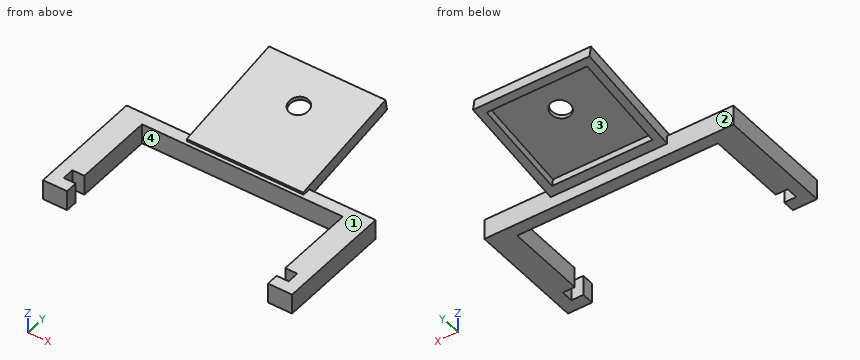
Autodesk Inventor part; units mm, degrees
ref_plane "YZ Plane" through (0, 0, 0) normal (1, 0, 0) x (0, 1, 0)
ref_plane "XZ Plane" through (0, 0, 0) normal (0, 1, 0) x (-1, 0, 0)
ref_plane "XY Plane" through (0, 0, 0) normal (0, 0, 1) x (1, 0, 0)
sketch "Esquisse1" plane through (0, 0, 0) normal (0, 0, 1) x (1, 0, 0)
  line L0 (-16.3902, 3.7398) -> (-19.3902, 3.7398)
  line L1 (-19.3902, 3.7398) -> (-19.3902, 0.7398)
  line L2 (-19.3902, 0.7398) -> (-16.3902, 0.7398)
  line L3 (-16.3902, 0.7398) -> (-16.3902, -2.2602)
  line L4 (-16.3902, -2.2602) -> (-22.3902, -2.2602)
  line L5 (-16.3902, 3.7398) -> (-16.3902, 23.7398)
  line L6 (33.6098, 23.7398) -> (33.6098, 3.7398)
  line L7 (33.6098, 3.7398) -> (36.6098, 3.7398)
  line L8 (36.6098, 3.7398) -> (36.6098, 0.7398)
  line L9 (36.6098, 0.7398) -> (33.6098, 0.7398)
  line L10 (33.6098, 0.7398) -> (33.6098, -2.2602)
  line L11 (33.6098, -2.2602) -> (39.6098, -2.2602)
  line L12 (-22.3902, 26.7398) -> (39.6098, 26.7398)
  line L13 (-16.3902, 23.7398) -> (33.6098, 23.7398)
  line L14 (-22.3902, 26.7398) -> (-22.3902, -2.2602)
  line L15 (39.6098, 26.7398) -> (39.6098, -2.2602)
  point P0 (0, 0)
  dimension "d0" = 56
  dimension "d1" = 3
  dimension "d2" = 3
  dimension "d3" = 3
  dimension "d4" = 3
  dimension "d5" = 20
  dimension "d6" = 20
  dimension "d7" = 50
  dimension "d8" = 3
  dimension "d9" = 6
  dimension "d10" = 6
  dimension "d11" = 3
  dimension "d12" = 3
extrude "Extrusion1" add sketch "Esquisse1" along normal blind 5
ref_plane "Plan de construction1" through (39.6098, 26.7398, 5) normal (0, 0.9848, 0.1736) x (-1, 0, 0)
sketch "Esquisse2" plane through (39.6098, 26.7398, 5) normal (0, 0.9848, 0.1736) x (-1, 0, 0)
  line L0 (45.5, -2) -> (16.5, -2)
  line L1 (16.5, -2) -> (16.5, 1)
  line L2 (16.5, 1) -> (45.5, 1)
  line L3 (45.5, 1) -> (45.5, -2)
  line L4 (0, 0) -> (62, 0)
  line L5 (0, -4.924) -> (0, 0)
  point P0 (39.6098, -0.2807)
  dimension "d16" = 29
  dimension "d17" = 3
  dimension "d18" = 1
  dimension "d23" = 16.5
extrude "Extrusion2" add sketch "Esquisse2" along normal blind 27 and the other way blind 2
sketch "Esquisse3" plane through (23.1098, 26.7398, 2.9691) normal (0, 0.1736, -0.9848) x (-1, 0, 0)
  line L0 (2, 25.3527) -> (27, 25.3527)
  line L1 (27, 25.3527) -> (27, 2.3527)
  line L2 (27, 2.3527) -> (2, 2.3527)
  line L3 (2, 2.3527) -> (2, 25.3527)
  line L4 (0, 27.3527) -> (29, 27.3527)
  line L5 (29, 0) -> (29, 27.3527)
  line L6 (-28.9, 0.3527) -> (57.9, 0.3527)
  line L7 (0, 0) -> (0, 27.3527)
  point P0 (23.1098, -26.8492)
  dimension "d24" = 2
  dimension "d25" = 2
  dimension "d26" = 2
  dimension "d27" = 2
extrude "Extrusion3" cut sketch "Esquisse3" against normal blind 2 contours L0 L1 L2 L3
sketch "Esquisse4" plane through (23.1098, 26.3925, 4.9388) normal (0, 0.1736, -0.9848) x (-1, 0, 0)
  circle A0 centre (14.3745, 17.1752) radius 2.5
  point P0 (23.1098, -26.8492)
  dimension "d30" = 5
extrude "Extrusion4" cut sketch "Esquisse4" against normal blind 10
properties part number "support_caméra"
Check sheet for the modelled part. Datum: model origin and axes. Units: mm. Face numbers are marked on the shaded views. Coordinates: 2 decimals unless noted, no trailing zeros. Loops run counter-clockwise (first coordinate to the right, second up) from the corner with the lowest first, then second, coordinate; pieces in that order, holes last. Notation, with made-up numbers: (-2.75, -19.75) -> (33.25, -19.75) arc R3 ccw to (33.25, -14.75) -> close; hole circle Ø10 at (-31.75, -26). An arc over 180 degrees is marked (long way). Write item = value, one per line. Start each with the question number.
1. Depth check by flat-ended pin: P1, Ø2.5, axis at x = 35, z = 3, coming from the +Y side; P2, Ø4, axis at y = 44, z = 7, coming from the -X side; P3, Ø2, axis at x = 11.5, y = 47, coming from the -Z side. Enter the tip coordinate at first touch or a pass-through.
2. Section check B-B on x = 20. Record the cut outline in (y, z), then the cut area to 3 significant figures.
3. Draft check along Y on the marked faces 1, 2, 3 and 4. Enter one of: released by +Y, released by -Y, zero draft, split by the parting line, or undercut.
4. Section check A-A on y = 2. Record the cut outline in (x, z).
5. Section check C-C on z = 1.5. Record the cut outline in (x, y).
6. Section check D-D on y = 48. Record the cut outline in (x, z).
7. Material ranges on line 1 (X direction, y = 50, z = 8.25); line 2 (X direction, y = 13, z = 2.25); line 3 (Y direction, x = -17, z = 3.5), recorded low to high.
Responses:
q1.P1 = 26.74
q1.P2 = -5.89
q1.P3 = 8.4
q2.outline = (23.74, 0) -> (26.74, 0) -> (26.74, 2.97) -> (29.06, 3.38) -> (28.71, 5.35) -> (51.36, 9.34) -> (51.71, 7.37) -> (53.68, 7.72) -> (53.16, 10.67) -> (24.6, 5.64) -> (24.71, 5) -> (23.74, 5) -> close
q2.area = 52.0 mm2
q3.face_1 = zero draft
q3.face_2 = released by +Y
q3.face_3 = undercut
q3.face_4 = released by -Y
q4.outline = (-22.39, 0) -> (-19.39, 0) -> (-19.39, 5) -> (-22.39, 5) -> close; (36.61, 0) -> (39.61, 0) -> (39.61, 5) -> (36.61, 5) -> close
q5.outline = (-22.39, -2.26) -> (-16.39, -2.26) -> (-16.39, 0.74) -> (-19.39, 0.74) -> (-19.39, 3.74) -> (-16.39, 3.74) -> (-16.39, 23.74) -> (33.61, 23.74) -> (33.61, 3.74) -> (36.61, 3.74) -> (36.61, 0.74) -> (33.61, 0.74) -> (33.61, -2.26) -> (39.61, -2.26) -> (39.61, 26.74) -> (-22.39, 26.74) -> close
q6.outline = (-5.89, 6.72) -> (-3.89, 6.72) -> (-3.89, 8.75) -> (21.11, 8.75) -> (21.11, 6.72) -> (23.11, 6.72) -> (23.11, 9.76) -> (-5.89, 9.76) -> close
q7.line_1 = -5.89 to -3.89, 21.11 to 23.11
q7.line_2 = -22.39 to -16.39, 33.61 to 39.61
q7.line_3 = -2.26 to 0.74, 3.74 to 26.74
